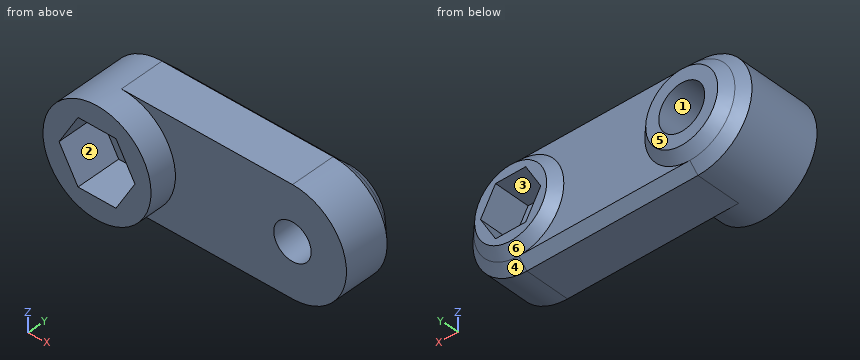
from build123d import *

# Parameters (mm, degrees)
EXTRUDE_1_DEPTH     = 10
CHAMFER_1_SIZE      = 2
CUT_EXTRUDE_1_DEPTH = 5
SKETCH_5_R          = 32.43595028
SKETCH_5_R_2        = 6
CUT_EXTRUDE_2_DEPTH = 3
CUT_EXTRUDE_3_DEPTH = 4
SKETCH_7_W          = 54.061660739
SKETCH_7_H          = 47.527586942
SKETCH_7_R          = 4
CUT_EXTRUDE_4_DEPTH = 1
CHAMFER_2_SIZE      = 1


with BuildPart() as part:
    # 草图1 → 凸台-拉伸1 (new body)
    with BuildSketch(Plane(origin=(0, 0, 0), x_dir=(1, 0, 0), z_dir=(0, 1, 0))):
        with BuildLine():
            Line((0, 6), (19, 6))
            ThreePointArc((19, 6), (25, 0), (19, -6))
            Line((19, -6), (0, -6))
            ThreePointArc((0, -6), (-6, 0), (0, 6))
        make_face()
    extrude(amount=EXTRUDE_1_DEPTH)

    # 草图2 → 切除-旋转1 (revolve, cut)
    with BuildSketch(Plane.XY, mode=Mode.PRIVATE) as cut_revolve_1_sk:
        Polygon((0, 10), (-2.55, 10), (-2.55, 5), (-1.6, 5), (-1.6, 2), (-2.55, 2), (-2.55, 0), (0, 0), align=None)
    revolve(cut_revolve_1_sk.sketch.rotate(Axis((0, -1.427566958, 0), (0, 1, 0)), 270), axis=Axis((0, -1.427566958, 0), (0, 1, 0)), mode=Mode.SUBTRACT)

    # 草图3 → 切除-旋转2 (revolve, cut)
    with BuildSketch(Plane.XY, mode=Mode.PRIVATE) as cut_revolve_2_sk:
        Polygon((19, 0), (16.925, 0), (16.925, 6), (16.5, 6), (16.5, 10), (19, 10), align=None)
    revolve(cut_revolve_2_sk.sketch.rotate(Axis((19, 0, 0), (0, 1, 0)), 270), axis=Axis((19, 0, 0), (0, 1, 0)), mode=Mode.SUBTRACT)

    # 倒角1
    chamfer_1_edges = [part.edges().sort_by_distance(p)[0] for p in [
        (25, 10, 0),
        (9.5, 10, -6),
        (-6, 10, 0),
        (9.5, 10, 6),
    ]]
    chamfer(chamfer_1_edges, length=CHAMFER_1_SIZE)

    # 草图4 → 切除-拉伸1 (cut)
    with BuildSketch(Plane.XZ):
        Polygon((2.107328483, 3.65), (-2.107328483, 3.65), (-4.214656965, 0), (-2.107328483, -3.65), (2.107328483, -3.65), (4.214656965, 0), align=None)
    extrude(amount=-CUT_EXTRUDE_1_DEPTH, mode=Mode.SUBTRACT)

    # 草图5 → 切除-拉伸2 (cut)
    with BuildSketch(Plane.XZ):
        Circle(SKETCH_5_R)
        with Locations(Location((0, 0, 0), (0, 0, 90))):
            Circle(SKETCH_5_R_2, mode=Mode.SUBTRACT)
    extrude(amount=-CUT_EXTRUDE_2_DEPTH, mode=Mode.SUBTRACT)

    # 草图6 → 切除-拉伸3 (cut)
    with BuildSketch(Plane(origin=(0, 10, 0), x_dir=(1, 0, 0), z_dir=(0, 1, 0))):
        Polygon((20.674315781, 2.9), (17.325684219, 2.9), (15.651368439, 0), (17.325684219, -2.9), (20.674315781, -2.9), (22.348631561, 0), align=None)
    extrude(amount=-CUT_EXTRUDE_3_DEPTH, mode=Mode.SUBTRACT)

    # 草图7 → 切除-拉伸4 (cut)
    with BuildSketch(Plane(origin=(0, 10, 0), x_dir=(1, 0, 0), z_dir=(0, 1, 0))):
        with Locations((6.682015694, 1.141108586)):
            Rectangle(SKETCH_7_W, SKETCH_7_H)
        with Locations(Location((0, 0, 0), (0, 0, 270))):
            Circle(SKETCH_7_R, mode=Mode.SUBTRACT)
        with Locations(Location((19, 0, 0), (0, 0, 270))):
            Circle(SKETCH_7_R, mode=Mode.SUBTRACT)
    extrude(amount=-CUT_EXTRUDE_4_DEPTH, mode=Mode.SUBTRACT)

    # 倒角2
    chamfer_2_edges = [part.edges().sort_by_distance(p)[0] for p in [
        (19, 9, -4),
        (0, 9, -4),
    ]]
    chamfer(chamfer_2_edges, length=CHAMFER_2_SIZE - 0.0001)  # a hair under: the kernel refuses the full size


solid = part.part
The model under review builds one solid part; all positions refer to its coordinate system, in mm. Face numbers are marked on the shaded views. A direction names the side the tool comes from. Round coordinates to 2 decimals unless told otherwise and drop trailing zeros. Order: outer loops, then holes, each group sorted by start corner. A loop starts at its lowest first (then second) coordinate and runs counter-clockwise, first axis right, second up. Notation, with made-up numbers: (58, 47) -> (94, 47) arc R25 cw to (94, 81) -> close; hole circle Ø8 at (81.25, 45). An arc over 180 degrees is marked (long way). Return JSON: item names as keys, results as strings.
1. Take a section at A-A (y = 8.5). Write out the cut boundary in (x, z).
Answer block:
{"outline": "(0, -5.5) -> (19, -5.5) arc R5.5 ccw to (19, 5.5) -> (0, 5.5) arc R5.5 ccw to start; hole circle Ø5.1 at (0, 0); hole (15.65, 0) -> (17.33, -2.9) -> (20.67, -2.9) -> (22.35, 0) -> (20.67, 2.9) -> (17.33, 2.9) -> close"}
2. Take a section at C-C (x = 10). Write out the cut boundary in (y, z).
Answer block:
{"outline": "(3, -6) -> (8, -6) -> (9, -5) -> (9, 5) -> (8, 6) -> (3, 6) -> close"}
3. The part is to be moulded in two halves that separate along X. For the marked faces 4, 5 and 6, say which applies: +X half, -X half, draft (parallel to the pull), parting line (faces both ways), or undercut.
Answer block:
{"face 4": "+X half", "face 5": "draft", "face 6": "undercut"}
4. Insertion check: P1, Ø3.5, axis at x = -1.5, z = 0.5, coming from the -Y side; P2, Ø1.5, axis at y = 6, z = -4, coming from the +X side; P3, Ø3, axis at x = 19, z = -2, coming from the -Y side. Each pin has a flat end and moves straight along its axis. Give the tip position at first contact, or say it passes through.
Answer block:
{"P1": "stops at y = 5", "P2": "stops at x = 24.04", "P3": "stops at y = 3"}
5. For L1, parallel to X at y = 5.1, z = 0 (3 decimals); L2, parallel to X at y = 5.75, z = 1; L3, parallel to Z at x = 19, y = 5.3 (3 decimals), list the stretches that pass through material, from the lowest coordinate up. Write a range as [from, to].
Answer block:
{"L1": "x = [-6, -2.55], [2.55, 16.925], [21.075, 25]", "L2": "x = [-5.92, -2.35], [2.35, 17.18], [20.82, 24.92]", "L3": "z = [-6, -2.075], [2.075, 6]"}
6. For the marked faces 1, 2 and 3, list the 3-axis set-ups (+Z, -Z, +X, -X, +Y, -Y) from which the entire face can be reached by the end or side of a thin tool; tool diameter is ignored.
Answer block:
{"face 1": "+Y, -Y", "face 2": "-Y", "face 3": "+Y"}
7. Take a section at B-B (x = 5.5). Write out the cut boundary in (y, z).
Answer block:
{"outline": "(0, -2.4) -> (3, -2.4) -> (3, -6) -> (8, -6) -> (9, -5) -> (9, 5) -> (8, 6) -> (3, 6) -> (3, 2.4) -> (0, 2.4) -> close"}
